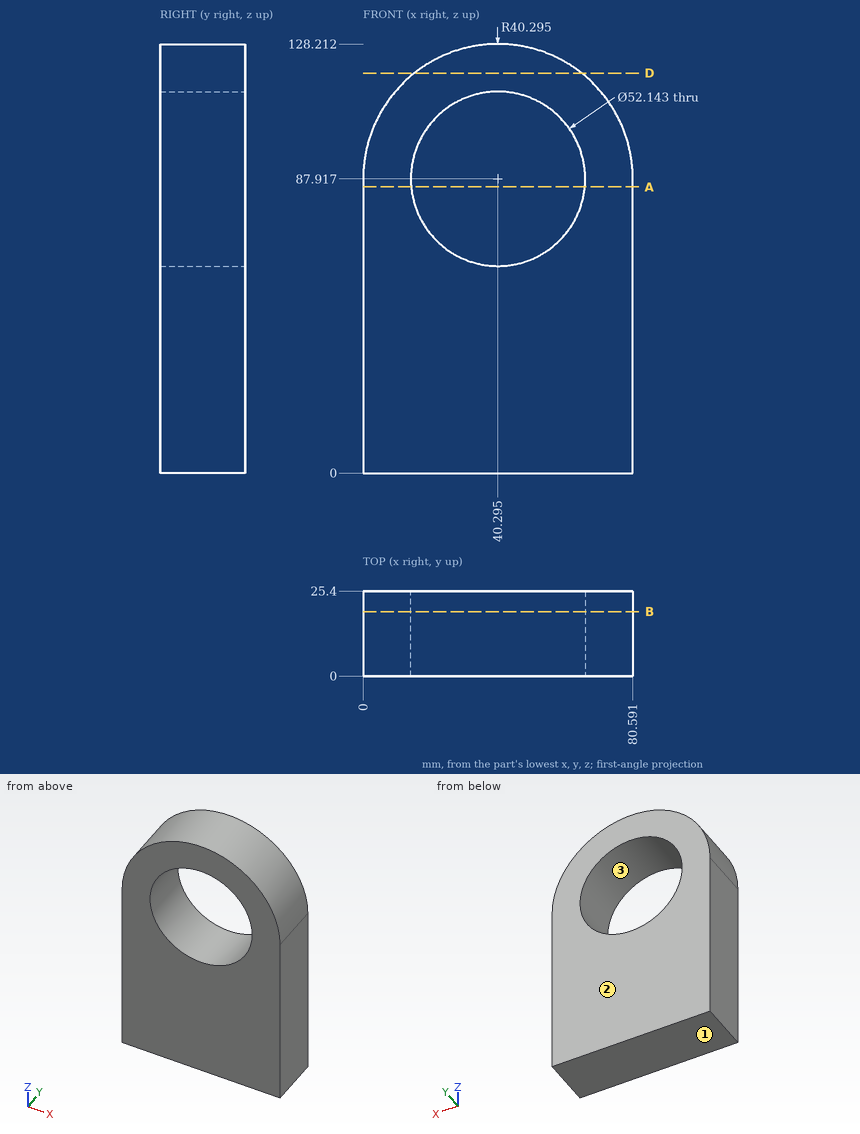
Drawing for the job (mm, zero at the part's lowest x, y, z). Give positions to 0.01 mm unless a question says otherwise; leave off trailing zeros. Order: outer loops, then holes, each group sorted by start corner. A loop starts at its lowest first (then second) coordinate and runs counter-clockwise, first axis right, second up. Notation, with made-up numbers: M 61.25,74 L 108.25,74 A21 cw 108.25,97 Z; hole C 59.5,24.5 d2. An arc over 180 degrees is marked long. Put each result on its own line as item: value. Start each with the question number.
(1) Saw through at A-A, the plane z = 85.5. Write the cut outline in (x, y) (1 decimal).
(2) Saw through at B-B, the plane y = 19.25. Write the cut outline in (x, z) (1 decimal), then the cut area to 3 significant figures.
(3) Saw through at D-D, the plane z = 119.5. Write the cut outline in (x, y), then the cut area to 3 significant figures.
(4) Flat gauge pin, fed straight in: pin 1 Ø1 at (y, z) = (5.5, 90) entering from -X. Where does the tip first touch, or does it go through?
(5) Drill centre lines: line 1 along X through (y, z) = (12, 87); line 2 along Z through (x, y) = (44, 10.75); line 3 along Z through (x, y) = (40, 11.5). Where is each one in solid material? Low to high.
(6) Mould opens along Z. For the marked faces 1, 2 and 3 say: +Z half, -Z half, draft (parallel to the pull), parting line (faces both ways), or undercut.
Check result:
1. outline: M 0,0 L 14.3,0 L 14.3,25.4 L 0,25.4 Z; M 66.3,0 L 80.6,0 L 80.6,25.4 L 66.3,25.4 Z
2. outline: M 0,0 L 80.6,0 L 80.6,87.9 A40.3 ccw 0,87.9 Z; hole C 40.3,87.9 d52.1
2. area: 7,500 mm2
3. outline: M 15.27,0 L 65.32,0 L 65.32,25.4 L 15.27,25.4 Z
3. area: 1,270 mm2
4. pin 1: stops at x = 0.03
5. line 1: x = 0 to 14.24, 66.35 to 80.59
5. line 2: z = 0 to 62.11, 113.72 to 128.04
5. line 3: z = 0 to 61.85, 113.99 to 128.21
6. face 1: -Z half
6. face 2: draft
6. face 3: undercut
